Geometry check sheet. Reference: the model listing, model coordinates, mm. A direction names the side the tool comes from. Coordinates: 2 decimals unless noted, no trailing zeros. Loops run counter-clockwise (first coordinate to the right, second up) from the corner with the lowest first, then second, coordinate; pieces in that order, holes last.
from build123d import *

# Parameters (mm, degrees)
SKETCH1_W           = 25
SKETCH1_H           = 12
SKETCH1_R           = 1.5
BOSS_EXTRUDE1_DEPTH = 0.7
SKETCH3_W           = 0.7
SKETCH3_H           = 12
BOSS_EXTRUDE3_DEPTH = 20
SKETCH4_R           = 2.15
CUT_EXTRUDE1_DEPTH  = 35.604768458


with BuildPart() as part:
    # Sketch1 → Boss-Extrude1 (new body)
    with BuildSketch(Plane(origin=(0, 0, 0), x_dir=(1, 0, 0), z_dir=(0, 1, 0))):
        with Locations((0, 6)):
            Rectangle(SKETCH1_W, SKETCH1_H)
        with Locations(Location((-5, 8, 0), (0, 0, 270))):
            Circle(SKETCH1_R, mode=Mode.SUBTRACT)
        with Locations(Location((5, 8, 0), (0, 0, 270))):
            Circle(SKETCH1_R, mode=Mode.SUBTRACT)
        with Locations(Location((0, 3.5, 0), (0, 0, 270))):
            Circle(SKETCH1_R, mode=Mode.SUBTRACT)
    extrude(amount=BOSS_EXTRUDE1_DEPTH)

    # Sketch3 → Boss-Extrude3 (add)
    with BuildSketch(Plane(origin=(0, 0.7, 0), x_dir=(1, 0, 0), z_dir=(0, 1, 0))):
        with Locations((-12.15, 6)):
            Rectangle(SKETCH3_W, SKETCH3_H)
    extrude(amount=BOSS_EXTRUDE3_DEPTH)

    # Sketch4 → Cut-Extrude1 (cut, through all)
    with BuildSketch(Plane.ZY.offset(12.5)):
        with Locations((-8, 5)):
            Circle(SKETCH4_R)
        with Locations((-8, 15)):
            Circle(SKETCH4_R)
    extrude(amount=-CUT_EXTRUDE1_DEPTH, mode=Mode.SUBTRACT)


solid = part.part
1) Mould release check, pull along Z, two halves, no side actions. Record for faces 3 (the flat face through (-5.6, 0.3, 0)), 4 (the cylindrical face through (-12.15, 6.81, -6.84)), 5 (the flat face through (0, 0.7, -6)): +Z half, -Z half, draft (parallel to the pull), parting line (faces both ways), or undercut.
Data:
face 3: +Z half
face 4: undercut
face 5: draft
2) Access from +Z, -Z, +X, -X, +Y, -Y to the whole of each face (thin tool, end or side, straight path). Record for faces 1 (the cylindrical face through (5.07, 0.35, -9.5)), 2 (the flat face through (-11.8, 11, -6)).
Data:
face 1: +Y, -Y
face 2: +Z, -Z, +X, +Y
3) Material ranges on probe 1 along X at (y, z) = (0.15, -8); probe 2 along Y at (x, z) = (-12.05, -8); probe 3 along Y at (x, z) = (3.25, -10.5), recorded low to high.
Data:
probe 1: x = -12.5 to -6.5, -3.5 to 3.5, 6.5 to 12.5
probe 2: y = 0 to 2.85, 7.15 to 12.85, 17.15 to 20.7
probe 3: y = 0 to 0.7
4) Section check B-B on y = 15. Record the cut outline in (x, z).
Data:
outline: (-12.5, -12) - (-11.8, -12) - (-11.8, -10.15) - (-12.5, -10.15) - close; (-12.5, -5.85) - (-11.8, -5.85) - (-11.8, 0) - (-12.5, 0) - close
5) Section check C-C on z = -8. Record the cut outline in (x, y), and give its area (3 significant figures).
Data:
outline: (-12.5, 0) - (-6.5, 0) - (-6.5, 0.7) - (-11.8, 0.7) - (-11.8, 2.85) - (-12.5, 2.85) - close; (-12.5, 7.15) - (-11.8, 7.15) - (-11.8, 12.85) - (-12.5, 12.85) - close; (-12.5, 17.15) - (-11.8, 17.15) - (-11.8, 20.7) - (-12.5, 20.7) - close; (-3.5, 0) - (3.5, 0) - (3.5, 0.7) - (-3.5, 0.7) - close; (6.5, 0) - (12.5, 0) - (12.5, 0.7) - (6.5, 0.7) - close
area: 21.3 mm2
6) Section check A-A on x = -5. Record the cut outline in (y, z), and give its area (3 significant figures).
Data:
outline: (0, -12) - (0.7, -12) - (0.7, -9.5) - (0, -9.5) - close; (0, -6.5) - (0.7, -6.5) - (0.7, 0) - (0, 0) - close
area: 6.30 mm2
7) Depth check by flat-ended pin: pin 1 (6 mm diameter, centred on x = -2, z = -8.5, fed in from +Y); pin 2 (2.5 mm diameter, centred on y = 15, z = -8, fed in from +X); pin 3 (3.5 mm diameter, centred on y = 9, z = -8.5, fed in from +X). Enter the tip coordinate at first touch or a pass-through.
Data:
pin 1: stops at y = 0.7
pin 2: passes through
pin 3: stops at x = -11.8
8) Section check D-D on z = -3.5. Record the cut outline in (x, y), and give its area (3 significant figures).
Data:
outline: (-12.5, 0) - (-1.5, 0) - (-1.5, 0.7) - (-11.8, 0.7) - (-11.8, 20.7) - (-12.5, 20.7) - close; (1.5, 0) - (12.5, 0) - (12.5, 0.7) - (1.5, 0.7) - close
area: 29.4 mm2
